Part print with two shaded views. Sizes in mm from the minimum x, y, z corner. Round coordinates to 2 decimals unless told otherwise and drop trailing zeros. Loops run counter-clockwise (first coordinate to the right, second up) from the corner with the lowest first, then second, coordinate; pieces in that order, holes last.
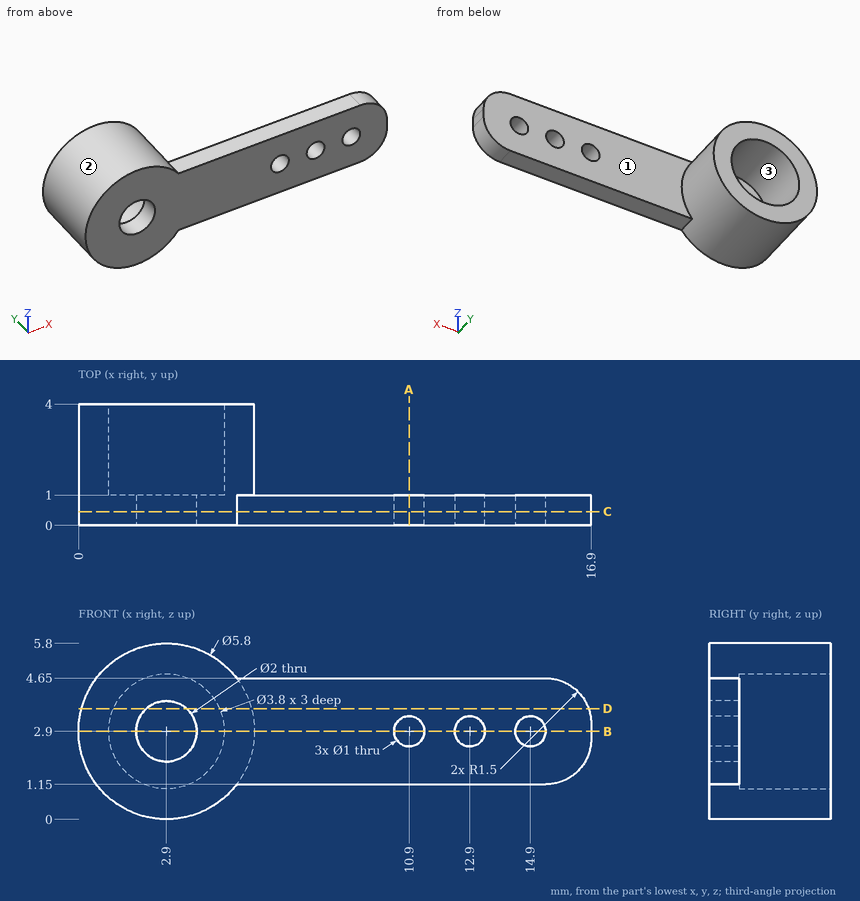
Item 1: Cut at D-D (z = 3.65). List the corners of the cut face in (x, y).
Verdict:
outline: (0.1, 0) - (2.24, 0) - (2.24, 1) - (1.15, 1) - (1.15, 4) - (0.1, 4) - close; (3.56, 0) - (16.81, 0) - (16.81, 1) - (5.7, 1) - (5.7, 4) - (4.65, 4) - (4.65, 1) - (3.56, 1) - close
Item 2: Mould opens along X. For the marked faces 1, 2 and 3 say: released by +X, released by -X, zero draft, split by the parting line, or undercut.
Verdict:
face 1: zero draft
face 2: split by the parting line
face 3: undercut
Item 3: Wall check: L1, parallel to X at y = 0.35, z = 2.9; L2, parallel to Z at x = 14.9, y = 0.7; L3, parallel to X at y = 3.3, z = 2.9. Give the ranges that are in metal, low to high.
Verdict:
L1: x = 0 to 1.9, 3.9 to 10.4, 11.4 to 12.4, 13.4 to 14.4, 15.4 to 16.9
L2: z = 1.15 to 2.4, 3.4 to 4.65
L3: x = 0 to 1, 4.8 to 5.8
Item 4: Cut at C-C (y = 0.45). List the corners of the cut face in (x, z), plus the area to 3 significant figures.
Verdict:
outline: (5.21, 1.15) - (15.4, 1.15) arc R1.5 ccw to (16.9, 2.65) - (16.9, 3.15) arc R1.5 ccw to (15.4, 4.65) - (5.21, 4.65) arc R2.9 ccw (long way) to start; hole circle Ø2 at (2.9, 2.9); hole circle Ø1 at (10.9, 2.9); hole circle Ø1 at (12.9, 2.9); hole circle Ø1 at (14.9, 2.9)
area: 59.5 mm2
Item 5: Cut at A-A (x = 10.9). List the corners of the cut face in (y, z).
Verdict:
outline: (0, 1.15) - (1, 1.15) - (1, 2.4) - (0, 2.4) - close; (0, 3.4) - (1, 3.4) - (1, 4.65) - (0, 4.65) - close
Item 6: Cut at B-B (z = 2.9). List the corners of the cut face in (x, y).
Verdict:
outline: (0, 0) - (1.9, 0) - (1.9, 1) - (1, 1) - (1, 4) - (0, 4) - close; (3.9, 0) - (10.4, 0) - (10.4, 1) - (5.8, 1) - (5.8, 4) - (4.8, 4) - (4.8, 1) - (3.9, 1) - close; (11.4, 0) - (12.4, 0) - (12.4, 1) - (11.4, 1) - close; (13.4, 0) - (14.4, 0) - (14.4, 1) - (13.4, 1) - close; (15.4, 0) - (16.9, 0) - (16.9, 1) - (15.4, 1) - close
Item 7: Flat gauge pins, fed straight in: P1, Ø3, axis at x = 2.9, z = 2.9, coming from the +Y side; P2, Ø0.8, axis at x = 11.5, y = 0.5, coming from the +Z side; P3, Ø0.8, axis at x = 11, y = 0.5, coming from the -Z side. Where does each tip first touch, or does it go through?
Verdict:
P1: stops at y = 1
P2: stops at z = 4.65
P3: stops at z = 1.15
